from build123d import *

# Parameters (mm, degrees)
PAD_DEPTH       = 2
PAD001_DEPTH    = 1.5
SKETCH002_R     = 4
PAD002_DEPTH    = 34
POCKET_DEPTH    = 8.001
SKETCH009_R     = 2
POCKET003_DEPTH = 5


with BuildPart() as part:
    # Sketch → Pad (new body)
    with BuildSketch(Plane.XY):
        with BuildLine():
            Line((-51.45, 35.75), (37.75, 35.75))
            ThreePointArc((41.75, 31.75), (40.578427, 34.578427), (37.75, 35.75))
            Line((41.75, 31.75), (41.75, -31.75))
            ThreePointArc((37.75, -35.75), (40.578427, -34.578427), (41.75, -31.75))
            Line((37.75, -35.75), (-51.45, -35.75))
            ThreePointArc((-55.45, -31.75), (-54.278427, -34.578427), (-51.45, -35.75))
            Line((-55.45, -31.75), (-55.45, 31.75))
            ThreePointArc((-51.45, 35.75), (-54.278427, 34.578427), (-55.45, 31.75))
        make_face()
        with BuildLine():
            Line((-26.75, -33.75), (26.75, -33.75))
            ThreePointArc((26.75, -33.75), (31.699747, -31.699747), (33.75, -26.75))
            Line((33.75, -26.75), (33.75, 26.75))
            ThreePointArc((33.75, 26.75), (31.699747, 31.699747), (26.75, 33.75))
            Line((26.75, 33.75), (-26.75, 33.75))
            ThreePointArc((-26.75, 33.75), (-31.699747, 31.699747), (-33.75, 26.75))
            Line((-33.75, 26.75), (-33.75, -26.75))
            ThreePointArc((-33.75, -26.75), (-31.699747, -31.699747), (-26.75, -33.75))
        make_face(mode=Mode.SUBTRACT)
    extrude(amount=PAD_DEPTH)

    # Sketch001 (on Face17 of Pad) → Pad001 (join)
    with BuildSketch(Plane(origin=(0, 0, 0), x_dir=(1, 0, 0), z_dir=(0, 0, -1))):
        with BuildLine():
            ThreePointArc((-51.45, 35.75), (-54.278427, 34.578427), (-55.45, 31.75))
            Line((-55.45, 31.75), (-55.45, -31.75))
            ThreePointArc((-55.45, -31.75), (-54.278427, -34.578427), (-51.45, -35.75))
            Line((37.75, -35.75), (-51.45, -35.75))
            ThreePointArc((37.75, -35.75), (40.578427, -34.578427), (41.75, -31.75))
            Line((41.75, 31.75), (41.75, -31.75))
            ThreePointArc((41.75, 31.75), (40.578427, 34.578427), (37.75, 35.75))
            Line((-51.45, 35.75), (37.75, 35.75))
        make_face()
        with BuildLine():
            ThreePointArc((-26.75, 31.75), (-30.285534, 30.285534), (-31.75, 26.75))
            Line((-31.75, -26.75), (-31.75, 26.75))
            ThreePointArc((-31.75, -26.75), (-30.285534, -30.285534), (-26.75, -31.75))
            Line((26.75, -31.75), (-26.75, -31.75))
            ThreePointArc((26.75, -31.75), (30.285534, -30.285534), (31.75, -26.75))
            Line((31.75, 26.75), (31.75, -26.75))
            ThreePointArc((31.75, 26.75), (30.285534, 30.285534), (26.75, 31.75))
            Line((-26.75, 31.75), (26.75, 31.75))
        make_face(mode=Mode.SUBTRACT)
    extrude(amount=PAD001_DEPTH)

    # Sketch002 (on Face5 of Pad001) → Pad002 (join)
    with BuildSketch(Plane.XY.offset(2)):
        with Locations((37.75, -31.75)):
            Circle(SKETCH002_R)
        with Locations((37.75, 16.65)):
            Circle(SKETCH002_R)
        with BuildLine():
            ThreePointArc((-51.45, 20.65), (-55.45, 16.65), (-51.45, 12.65))
            Line((-51.45, 12.65), (-41.25, 12.65))
            ThreePointArc((-41.25, 12.65), (-37.25, 16.65), (-41.25, 20.65))
            Line((-41.25, 20.65), (-51.45, 20.65))
        make_face()
        with BuildLine():
            ThreePointArc((-41.25, -35.75), (-37.25, -31.75), (-41.25, -27.75))
            Line((-41.25, -27.75), (-51.45, -27.75))
            ThreePointArc((-51.45, -27.75), (-55.45, -31.75), (-51.45, -35.75))
            Line((-51.45, -35.75), (-41.25, -35.75))
        make_face()
    extrude(amount=PAD002_DEPTH)

    # Sketch003 (on Face16 of Pad002) → Pocket (cut, through all)
    with BuildSketch(Plane(origin=(0, -27.75, 0), x_dir=(-1, 0, 0), z_dir=(0, 1, 0))):
        with BuildLine():
            ThreePointArc((43.6, 12), (46.35, 9.25), (49.1, 12))
            Line((49.1, 12), (49.1, 17))
            ThreePointArc((49.1, 17), (46.35, 19.75), (43.6, 17))
            Line((43.6, 17), (43.6, 12))
        make_face()
    extrude(amount=-POCKET_DEPTH, mode=Mode.SUBTRACT)

    # Sketch009 (on Face33 of Pocket) → Pocket003 (cut)
    with BuildSketch(Plane.XY.offset(36)):
        with Locations((-51.45, 16.65)):
            Circle(SKETCH009_R)
        with Locations((-41.25, 16.65)):
            Circle(SKETCH009_R)
        with Locations((37.75, 16.65)):
            Circle(SKETCH009_R)
        with Locations((37.75, -31.75)):
            Circle(SKETCH009_R)
        with Locations((-41.25, -31.75)):
            Circle(SKETCH009_R)
        with Locations((-51.45, -31.75)):
            Circle(SKETCH009_R)
    extrude(amount=-POCKET003_DEPTH, mode=Mode.SUBTRACT)


solid = part.part
Could you check a few things on this model? Use its own coordinates, in mm. A direction names the side the tool comes from. Round coordinates to 2 decimals unless told otherwise and drop trailing zeros. Write each loop counter-clockwise with the first axis right and the second up, starting at its lowest first coordinate (ties: lowest second). Pieces come first, ordered by that corner, then holes. Notation, with made-up numbers: (3, 64.25) -> (12, 64.25) arc R26 cw to (12, 79.25) -> close; hole circle Ø7 at (40.25, 61). An arc over 180 degrees is marked (long way). Use a Markdown table: item, result.
1. If we section it at A-A (z = 7.5): List the corners of the cut face in (x, y) for me, then the cut area to 3 significant figures.
Answer key:
| item | result |
|---|---|
| outline | (-51.45, -35.75) -> (-41.25, -35.75) arc R4 ccw to (-41.25, -27.75) -> (-51.45, -27.75) arc R4 ccw to start; (-51.45, 12.65) -> (-41.25, 12.65) arc R4 ccw to (-41.25, 20.65) -> (-51.45, 20.65) arc R4 ccw to start; circle Ø8 at (37.75, -31.75); circle Ø8 at (37.75, 16.65) |
| area | 364 mm^2 |
2. If we section it at C-C (y = 23): List the corners of the cut face in (x, z) for me, then the cut area to 3 significant figures.
Answer key:
| item | result |
|---|---|
| outline | (-55.45, -1.5) -> (-31.75, -1.5) -> (-31.75, 0) -> (-33.75, 0) -> (-33.75, 2) -> (-55.45, 2) -> close; (31.75, -1.5) -> (41.75, -1.5) -> (41.75, 2) -> (33.75, 2) -> (33.75, 0) -> (31.75, 0) -> close |
| area | 110 mm^2 |
3. For pin 1 Ø5 at (x, z) = (-46.5, 26.5) entering from +Y; pin 2 Ø3 at (x, z) = (-37, 31) entering from +Y; pin 3 Ø8 at (x, y) = (-35.5, 8) entering from +Z, each with a flat end and sliding along its axis, tell me the tip position at first contact or that it passes through.
Answer key:
| item | result |
|---|---|
| pin 1 | stops at y = 20.65 |
| pin 2 | stops at y = 19.55 |
| pin 3 | stops at z = 2 |
4. Please list where these lines run through material, in increasing order: probe 1 along Y at (x, z) = (37.75, 34.9); probe 2 along X at (y, z) = (-32, 5).
Answer key:
| item | result |
|---|---|
| probe 1 | y = -35.75 to -33.75, -29.75 to -27.75, 12.65 to 14.65, 18.65 to 20.65 |
| probe 2 | x = -55.44 to -37.26, 33.76 to 41.74 |
5. We'd pull the mould along Y, two halves only. Please class faces 1 (the face through (-30.32, 30.25, -0.74)), 2 (the face through (-51, 17, 31)), 3 (the face through (-46, 20.65, 19)), 4 (the face through (-40, -8, -1.5)): +Y half, -Y half, draft (parallel to the pull), parting line (faces both ways), or undercut.
Answer key:
| item | result |
|---|---|
| face 1 | undercut |
| face 2 | undercut |
| face 3 | +Y half |
| face 4 | draft |
6. If we section it at D-D (x = -46.35): List the corners of the cut face in (y, z) for me.
Answer key:
| item | result |
|---|---|
| outline | (-35.75, -1.5) -> (35.75, -1.5) -> (35.75, 2) -> (20.65, 2) -> (20.65, 36) -> (12.65, 36) -> (12.65, 2) -> (-27.75, 2) -> (-27.75, 9.25) -> (-35.75, 9.25) -> close; (-35.75, 19.75) -> (-27.75, 19.75) -> (-27.75, 36) -> (-35.75, 36) -> close |
7. Which directions (+Z, -Z, +X, -X, +Y, -Y) give clear straight access to the entire face, cutting with the end or side of a thin tool? Please do faces 5 (the face through (-55.45, 16.74, 18.76)), 6 (the face through (-41, -32, 31)), 7 (the face through (30.25, 30.32, -0.74)), 8 (the face through (-49.1, -32, 14)).
Answer key:
| item | result |
|---|---|
| face 5 | +Z, -X |
| face 6 | +Z |
| face 7 | +Z, -Z |
| face 8 | -Y |
8. If we section it at B-B (x = -12.5): List the corners of the cut face in (y, z) for me.
Answer key:
| item | result |
|---|---|
| outline | (-35.75, -1.5) -> (-31.75, -1.5) -> (-31.75, 0) -> (-33.75, 0) -> (-33.75, 2) -> (-35.75, 2) -> close; (31.75, -1.5) -> (35.75, -1.5) -> (35.75, 2) -> (33.75, 2) -> (33.75, 0) -> (31.75, 0) -> close |
